Check sheet for the modelled part. Datum: model origin and axes. Units: mm. A direction names the side the tool comes from. Give positions to 0.01 mm unless a question says otherwise; leave off trailing zeros. Order: outer loops, then holes, each group sorted by start corner. A loop starts at its lowest first (then second) coordinate and runs counter-clockwise, first axis right, second up. Notation, with made-up numbers: (87, -32.75) -> (116, -32.75) arc R31 ccw to (116, 3.25) -> close; hole circle Ø9 at (82, 49.25). An arc over 180 degrees is marked (long way). One line per question, with ' | ' between items. Start each with the question number.
Autodesk Inventor part; units mm, degrees
ref_plane "YZ Plane" through (0, 0, 0) normal (1, 0, 0) x (0, 1, 0)
ref_plane "XZ Plane" through (0, 0, 0) normal (0, 1, 0) x (-1, 0, 0)
ref_plane "XY Plane" through (0, 0, 0) normal (0, 0, 1) x (1, 0, 0)
sketch "Sketch1" plane through (0, 0, 0) normal (0, 1, 0) x (-1, 0, 0)
  line L0 (0, 0) -> (70, 0)
  line L1 (70, 0) -> (70, -150)
  line L2 (70, -150) -> (0, -150)
  line L3 (0, -150) -> (0, 0)
  dimension "d0" = 70
  dimension "d1" = 150
extrude "Plate1" add sketch "Sketch1" along normal blind 5
sketch "Sketch2" plane through (0, 0, -150) normal (0, 0, -1) x (-1, 0, 0)
  line L0 (70, 5) -> (0, 5)
  line L1 (0, 5) -> (70, 5)
  line L2 (70, 5) -> (70, -36)
  line L3 (70, -36) -> (0, -36)
  line L4 (0, -36) -> (0, 5)
  point P0 (0, 0)
  dimension "d3" = 70
  dimension "d4" = 41
sheet face with bend "Face2" sketch "Sketch2" thickness 5 toward (0, 0, -1) bend radius 5
bend "Bend1"
sketch "Sketch3" plane through (0, 0, -155) normal (0, 0, -1) x (-1, 0, 0)
  line L0 (70, -36) -> (0, -36)
  line L1 (70, -5) -> (70, -36)
  point P0 (0, 0)
  point P1 (45, -18)
  point P2 (15, -18)
  dimension "d10" = 18
  dimension "d11" = 18
  dimension "d19" = 25
  dimension "d20" = 30
hole "Hole1" at (-45, -18, -155) at (-15, -18, -155) direction (0, 0, 1) diameter 4.134 depth 5
sketch "Sketch4" plane through (0, 5, 0) normal (0, 1, 0) x (1, 0, 0)
  line L0 (-70, 145) -> (0, 145)
  line L1 (-55, 145) -> (-55, 0) construction
  line L2 (-70, 0) -> (0, 0)
  line L3 (-70, 0) -> (-70, 145)
  line L4 (-57.25, 131) -> (-52.75, 131)
  line L5 (-52.75, 131) -> (-52.75, 140)
  line L6 (-52.75, 140) -> (-57.25, 140)
  line L7 (-57.25, 140) -> (-57.25, 131)
  line L8 (-57.25, 131) -> (-52.75, 140) construction
  line L9 (-52.75, 131) -> (-57.25, 140) construction
  arc A0 (-52.75, 140) -> (-57.25, 140) centre (-55, 140) ccw
  arc A1 (-57.25, 131) -> (-52.75, 131) centre (-55, 131) ccw
  line L10 (-55, 140) -> (-51.5, 76.0958) construction
  line L11 (-55, 140) -> (9, 140) construction
  line L12 (-55, 131) -> (-51.5, 67.0958) construction
  line L13 (-55, 131) -> (9, 131) construction
  line L14 (-58.5, 67) -> (-51.5, 67)
  line L15 (-51.5, 67) -> (-51.5, 76)
  line L16 (-51.5, 76) -> (-58.5, 76)
  line L17 (-58.5, 76) -> (-58.5, 67)
  line L18 (-58.5, 67) -> (-51.5, 76) construction
  line L19 (-51.5, 67) -> (-58.5, 76) construction
  arc A2 (-51.5, 76) -> (-58.5, 76) centre (-55, 76) ccw
  arc A3 (-58.5, 67) -> (-51.5, 67) centre (-55, 67) ccw
  point P0 (-70, 72.5)
  point P1 (-55, 135.5)
  point P2 (-55, 71.5)
  dimension "d21" = 15
  dimension "d22" = 4.5
  dimension "d23" = 9
  dimension "d25" = 5
  dimension "d32" = 64
  dimension "d34" = 64
  dimension "d36" = 7
  dimension "d37" = 9
  dimension "d40" = 64
extrude "Extrusion1" cut sketch "Sketch4" against normal up to surface (5 mm away)
sketch "Sketch5" plane through (0, 5, 0) normal (0, 1, 0) x (1, 0, 0)
  line L0 (-70, 0) -> (-70, 145)
  line L1 (0, 0) -> (-70, 0)
  point P0 (-17.3, 42)
  point P1 (-17.3, 12)
  dimension "d41" = 52.7
  dimension "d42" = 52.7
  dimension "d50" = 30
  dimension "d51" = 12
hole "Hole2" at (-17.3, 5, -12) at (-17.3, 5, -42) direction (0, -1, 0) diameter 8.5 end through all
equation "\"d17\" = Thickness"
equation "\"d37\" = d23"
equation "\"d2\" = Thickness"
equation "\"d5\" = BendRadius"
equation "\"d6\" = BendReliefWidth"
equation "\"d8\" = MinimumRemnant"
equation "\"d7\" = BendReliefDepth"
equation "\"d9\" = TransitionRadius"
equation "\"BendRadius\" = Thickness"
equation "\"BendReliefWidth\" = Thickness"
equation "\"BendReliefDepth\" = 0.5 * Thickness"
equation "\"TransitionRadius\" = BendRadius"
equation "\"JacobiRadiusSize\" = BendRadius"
equation "\"GapSize\" = Thickness"
properties part number "ER_Halterung_Kantensensor"
1. Cross-section at D-D on x = -55. Record the boundary of the cut face in (y, z), and give its area (3 significant figures).
2. Go/stop test with flat-tipped pins: pin 1 (3.5 mm diameter, centred on x = -15, y = -18, fed in from -Z); pin 2 (2 mm diameter, centred on x = -33, y = -9.5, fed in from +Z); pin 3 (10 mm diameter, centred on x = -17.3, z = -42, fed in from -Y); pin 4 (2 mm diameter, centred on x = -13, y = -2, fed in from +Z). Record where each tip stops, or that it passes through.
3. Cross-section at A-A on z = -42. Record the boundary of the cut face in (x, y).
4. Cross-section at C-C on x = -45. Record the boundary of the cut face in (y, z).
5. Tool access check on faces 1 (the face through (-35, 5, -71)), 2 (the face through (-35, -20, -150)), 3 (the face through (-57.25, 3, -136)). Record the directions out of +Z, -Z, +X, -X, +Y, -Y that give a thin tool (end or side, any length) a straight path to the whole face; none if there is none.
6. Cross-section at B-B on y = -18. Record the boundary of the cut face in (x, z), and give its area (3 significant figures).
7. Mould release check, pull along Z, two halves, no side actions. Record for faces 4 (the face through (-51.5, 3, -71)), 5 (the face through (-35, -20, -155)), 6 (the face through (-35, 2, 0)): +Z half, -Z half, draft (parallel to the pull), parting line (faces both ways), or undercut.
8. Scan lines: probe 1 along X at (y, z) = (2, -12); probe 2 along Z at (x, y) = (-17.3, 1.45); probe 3 along Y at (x, z) = (-63, -109.5). Record each from-to range of solid material in increasing order.
Response values:
1) outline: (-36, -155) -> (-5, -155) arc R10 ccw to (5, -145) -> (5, -142.25) -> (0, -142.25) -> (0, -145) arc R5 cw to (-5, -150) -> (-36, -150) -> close; (0, -128.75) -> (5, -128.75) -> (5, -79.5) -> (0, -79.5) -> close; (0, -63.5) -> (5, -63.5) -> (5, 0) -> (0, 0) -> close | area: 791 mm²
2) pin 1: passes through | pin 2: stops at z = -150 | pin 3: stops at y = 0 | pin 4: stops at z = -148
3) outline: (-70, 0) -> (-21.55, 0) -> (-21.55, 5) -> (-70, 5) -> close; (-13.05, 0) -> (0, 0) -> (0, 5) -> (-13.05, 5) -> close
4) outline: (-36, -155) -> (-20.07, -155) -> (-20.07, -150) -> (-36, -150) -> close; (-15.93, -155) -> (-5, -155) arc R10 ccw to (5, -145) -> (5, 0) -> (0, 0) -> (0, -145) arc R5 cw to (-5, -150) -> (-15.93, -150) -> close
5) face 1: +Z, -Z, +X, -X, +Y | face 2: +Z, +X, -X, -Y | face 3: +Y, -Y
6) outline: (-70, -155) -> (-47.07, -155) -> (-47.07, -150) -> (-70, -150) -> close; (-42.93, -155) -> (-17.07, -155) -> (-17.07, -150) -> (-42.93, -150) -> close; (-12.93, -155) -> (0, -155) -> (0, -150) -> (-12.93, -150) -> close | area: 309 mm²
7) face 4: undercut | face 5: -Z half | face 6: +Z half
8) probe 1: x = -70 to -21.55, -13.05 to 0 | probe 2: z = -152.64 to -46.25, -37.75 to -16.25, -7.75 to 0 | probe 3: y = 0 to 5
